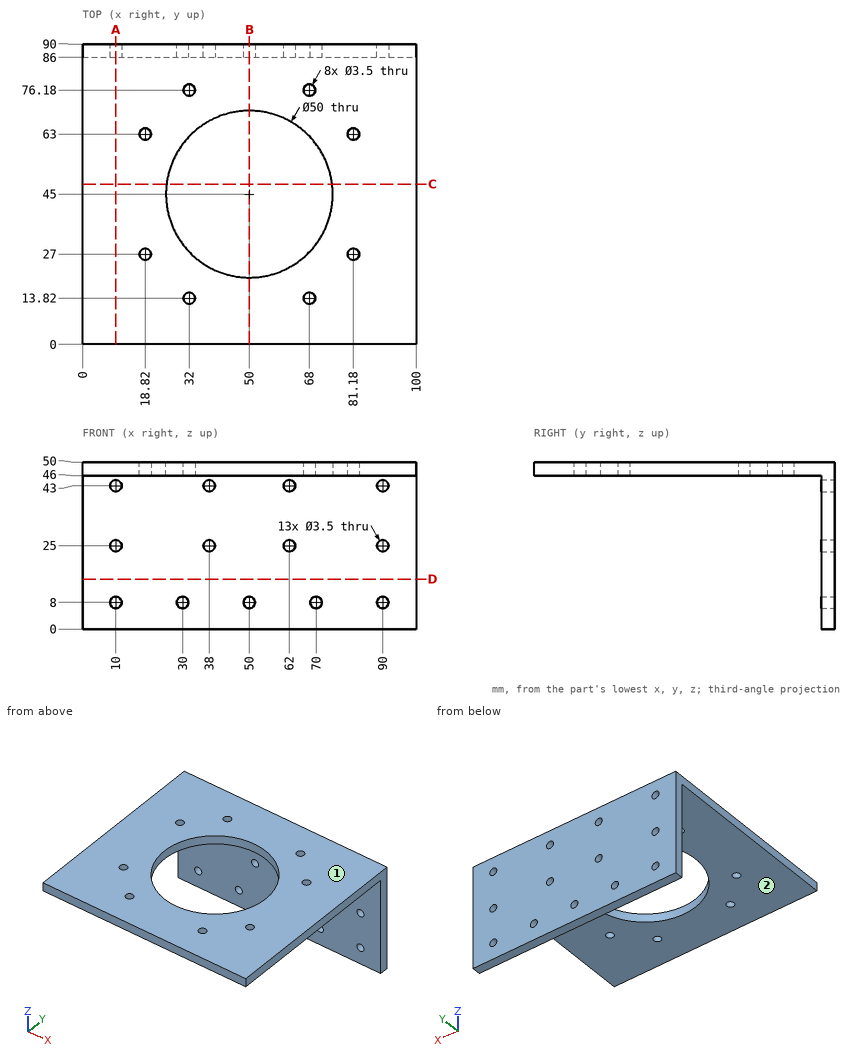
Input: dimensioned drawing with shaded views. Units: mm. Origin: part minimum x, y, z. A direction names the side the tool comes from. Give positions to 0.01 mm unless a question says otherwise; leave off trailing zeros. Order: outer loops, then holes, each group sorted by start corner. A loop starts at its lowest first (then second) coordinate and runs counter-clockwise, first axis right, second up.
(1) Contact query for flat-ended pins moving along their axis: P1, Ø4, axis at x = 81.18, y = 27, coming from the -Z side; P2, Ø4.5, axis at x = 62, z = 43, coming from the -Y side; P3, Ø3, axis at x = 68, y = 13.82, coming from the -Z side. Output: stop coordinate, or through.
(2) Access query for the marked faces 1 and 2. Directions: +Z, -Z, +X, -X, +Y, -Y. A direction counts if a zero-diameter tool reaches every point of the face in a straight line with its end or side. Return the directions, or none.
(3) Section query B-B (x = 50). Return the cut outline in (y, z).
(4) Section query A-A (x = 10). Return the cut outline in (y, z).
(5) Section query D-D (z = 15). Return the cut outline in (x, y), plus the area to 3 significant figures.
(6) Section query C-C (y = 48). Return the cut outline in (x, z), plus the area to 3 significant figures.
(7) Material intervals for line 1 along X through (y, z) = (13.82, 48.9); line 2 along X through (y, z) = (88.4, 8); line 3 along Y through (x, z) = (21, 23), sorted ascending.
Outcome:
1. P1: stops at z = 46
1. P2: stops at y = 86
1. P3: passes through
2. face 1: +Z, +X, -X, +Y, -Y
2. face 2: -Z, +X, -X, -Y
3. outline: (0, 46) - (20, 46) - (20, 50) - (0, 50) - close; (70, 46) - (86, 46) - (86, 9.75) - (90, 9.75) - (90, 50) - (70, 50) - close; (86, 0) - (90, 0) - (90, 6.25) - (86, 6.25) - close
4. outline: (0, 46) - (86, 46) - (86, 44.75) - (90, 44.75) - (90, 50) - (0, 50) - close; (86, 0) - (90, 0) - (90, 6.25) - (86, 6.25) - close; (86, 9.75) - (90, 9.75) - (90, 23.25) - (86, 23.25) - close; (86, 26.75) - (90, 26.75) - (90, 41.25) - (86, 41.25) - close
5. outline: (0, 86) - (100, 86) - (100, 90) - (0, 90) - close
5. area: 400 mm2
6. outline: (0, 46) - (25.18, 46) - (25.18, 50) - (0, 50) - close; (74.82, 46) - (100, 46) - (100, 50) - (74.82, 50) - close
6. area: 201 mm2
7. line 1: x = 0 to 30.25, 33.75 to 66.25, 69.75 to 100
7. line 2: x = 0 to 8.25, 11.75 to 28.25, 31.75 to 48.25, 51.75 to 68.25, 71.75 to 88.25, 91.75 to 100
7. line 3: y = 86 to 90
